Check sheet for the modelled part. Datum: model origin and axes. Units: mm. A direction names the side the tool comes from. Round coordinates to 2 decimals unless told otherwise and drop trailing zeros. Loops run counter-clockwise (first coordinate to the right, second up) from the corner with the lowest first, then second, coordinate; pieces in that order, holes last. Notation, with made-up numbers: M 44,-23 L 69,-23 A17 ccw 69,-10 Z; hole C 24,16 d10. An arc over 180 degrees is marked long. One line per question, with ' | ' between items. Start each with the question number.
(1) Section check B-B (y = 2.25). Record the boundary of the cut face in (x, z) (3 decimals).
(2) Section check A-A (x = 0). Record the boundary of the cut face in (y, z) (3 decimals), and give its area (3 significant figures).
(3) Section check C-C (x = -19). Record the boundary of the cut face in (y, z), and give its area (3 significant figures).
(4) Section check D-D (y = -8). Record the boundary of the cut face in (x, z), and give its area (3 significant figures).
(5) Go/stop test with a flat-tipped pin: P1, Ø10, axis at x = 16.5, y = -8, coming from the +Z side. Record where the tip stops, or that it passes through.
(6) Tool access check on faces 1 (the face through (0, 0, -12.7)), 2 (the face through (0.61, -4.66, 4.7)). Record the directions out of +Z, -Z, +X, -X, +Y, -Y that give a thin tool (end or side, any length) a straight path to the whole face; none if there is none.
(7) Thickness scan on probe 1 along Z at (x, y) = (18.5, -4); probe 2 along Y at (x, z) = (0, 1.5); probe 3 along Y at (x, z) = (-4, 7). Record the ranges inside material, lowest first. Write a range as [from, to].
```python
from build123d import *

# Parameters (mm, degrees)
SKETCH2_W           = 43.18
SKETCH2_H           = 25.4
BOSS_EXTRUDE3_DEPTH = 12.7
SKETCH4_R           = 4.699
BOSS_EXTRUDE4_DEPTH = 9.525


with BuildPart() as part:
    # Sketch2 → Boss-Extrude3 (new body)
    with BuildSketch(Plane.XY):
        Rectangle(SKETCH2_W, SKETCH2_H)
    extrude(amount=-BOSS_EXTRUDE3_DEPTH)

    # Sketch4 → Boss-Extrude4 (add)
    with BuildSketch(Plane.XY):
        with Locations(Location((0, 0, 0), (0, 0, 180))):
            Circle(SKETCH4_R)
    extrude(amount=BOSS_EXTRUDE4_DEPTH)


solid = part.part
```
The answers:
1) outline: M -21.59,-12.7 L 21.59,-12.7 L 21.59,0 L 4.125,0 L 4.125,9.525 L -4.125,9.525 L -4.125,0 L -21.59,0 Z
2) outline: M -12.7,-12.7 L 12.7,-12.7 L 12.7,0 L 4.699,0 L 4.699,9.525 L -4.699,9.525 L -4.699,0 L -12.7,0 Z | area: 412 mm²
3) outline: M -12.7,-12.7 L 12.7,-12.7 L 12.7,0 L -12.7,0 Z | area: 323 mm²
4) outline: M -21.59,-12.7 L 21.59,-12.7 L 21.59,0 L -21.59,0 Z | area: 548 mm²
5) P1: z = 0
6) face 1: -Z, +X, -X, +Y, -Y | face 2: +Z
7) probe 1: [-12.7, 0] | probe 2: [-4.7, 4.7] | probe 3: [-2.47, 2.47]
